Read the model definition and answer for the solid it produces. Units are mm, in the model's axes. A direction names the side the tool comes from. Give positions to 0.01 mm unless a question says otherwise; leave off trailing zeros. Loops run counter-clockwise (first coordinate to the right, second up) from the corner with the lowest first, then second, coordinate; pieces in that order, holes last. Notation, with made-up numbers: (87.5, -24.5) -> (97.5, -24.5) arc R27 ccw to (97.5, -0.5) -> close; hole circle Ø9 at (-24, -26.75). An arc over 180 degrees is marked (long way). Return JSON: item names as keys, results as strings. Group by question number.
Autodesk Inventor part; units mm, degrees
ref_plane "YZ Plane" through (0, 0, 0) normal (1, 0, 0) x (0, 1, 0)
ref_plane "XZ Plane" through (0, 0, 0) normal (0, 1, 0) x (-1, 0, 0)
ref_plane "XY Plane" through (0, 0, 0) normal (0, 0, 1) x (1, 0, 0)
sketch "Skizze1" plane through (0, 0, 0) normal (0, 0, 1) x (1, 0, 0)
  line L0 (0, 10) -> (50, 10)
  line L1 (50, 10) -> (50, -45)
  line L2 (50, -45) -> (0, -45)
  line L3 (0, -45) -> (-5, -45)
  line L4 (-5, -45) -> (-5, 10)
  line L5 (-5, 10) -> (0, 10)
  point P0 (0, 0)
  dimension "d0" = 10
  dimension "d1" = 50
  dimension "d2" = 55
  dimension "d3" = 50
  dimension "d6" = 5
extrude "Extrusion1" add sketch "Skizze1" along normal blind 3
sketch "Skizze3" plane through (0, 0, 3) normal (0, 0, 1) x (1, 0, 0)
  line L0 (50, 10) -> (-5, 10)
  line L1 (-5, 10) -> (-5, -45)
  line L2 (-5, 10) -> (-2, 10)
  line L3 (-2, 10) -> (-2, -45)
  line L4 (-5, -45) -> (50, -45)
  line L5 (-5, -45) -> (-5, 10)
  point P0 (0, 0)
  dimension "d13" = 3
extrude "Extrusion3" add sketch "Skizze3" along normal blind 20
fillet "Rundung2" radius 2 2 edges at (-2, -17.5, 3) (-5, -17.5, 0)
sketch "Skizze4" plane through (0, 0, 3) normal (0, 0, 1) x (1, 0, 0)
  circle A0 centre (46, -36.5) radius 3
  circle A1 centre (4, 6) radius 3
  circle A2 centre (4, 6) radius 1.8
  circle A3 centre (46, -36.5) radius 1.8
  point P0 (0, 0)
  dimension "d17" = 3.6
  dimension "d18" = 6
hole "Bohrung1" at (4, 6, 3) at (46, -36.5, 3) direction (0, 0, -1) diameter 6 end through all counterbore diameter 7 counterbore depth 1
properties part number "stativ"
1. Determine the mould class of faces 4 (the cylindrical face through (-1.43, -17.89, 3.6)), 5 (the flat face through (23, -17, 0)), 6 (the cylindrical face through (43.97, -34.29, 0.99)) for opening direction X: pulls with the +X half, pulls with the -X half, needs draft (parallel to the pull), parting line crosses it, or undercut.
2. Flat-ended cylindrical pins translate along their axes: pin 1 Ø4 at (x, y) = (4, 6) entering from -Z; pin 2 Ø3 at (x, y) = (8.5, -1) entering from +Z; pin 3 Ø2 at (y, z) = (-33.5, 6) entering from +X. Find the tip coordinate at first contact, or state that the pin passes through.
3. Section C-C on y = -20 is taken. Determine the outline of the cut face in (x, z), then the cut area to 3 significant figures.
4. Section B-B on x = 4 is taken. Determine the outline of the cut face in (y, z), then the cut area to 3 significant figures.
5. Straight lines are drawn through the part: line 1 (Y direction, x = 46, z = 2.5); line 2 (Y direction, x = 46, z = 0.6); line 3 (X direction, y = 6, z = 2.55). For each, find the intervals that lie inside material, in ascending order. Write a range as from..to.
6. Section D-D on z = 9.75 is taken. Determine the outline of the cut face in (x, y).
7. Section A-A on y = 6 is taken. Determine the outline of the cut face in (x, z).
8. Which of the six approach directions +Z, -Z, +X, -X, +Y, -Y give full straight-line access (tool end or side, diameter ignored) to faces 1 (the cylindrical face through (-4.4, -17.11, 0.57)), 2 (the flat face through (-2, -17, 14)), 3 (the flat face through (44, -39, 2))?
Completed:
{
 "1": {"face 4": "pulls with the +X half", "face 5": "needs draft", "face 6": "undercut"},
 "2": {"pin 1": "passes through", "pin 2": "stops at z = 3", "pin 3": "stops at x = -2"},
 "3": {"outline": "(-5, 2) arc R2 ccw to (-3, 0) -> (50, 0) -> (50, 3) -> (0, 3) arc R2 cw to (-2, 5) -> (-2, 23) -> (-5, 23) -> close", "area": "225 mm²"},
 "4": {"outline": "(-45, 0) -> (3, 0) -> (3, 2) -> (2.5, 2) -> (2.5, 3) -> (-45, 3) -> close; (9, 0) -> (10, 0) -> (10, 3) -> (9.5, 3) -> (9.5, 2) -> (9, 2) -> close", "area": "146 mm²"},
 "5": {"line 1": "y = -45..-40, -33..10", "line 2": "y = -45..-39.5, -33.5..10", "line 3": "x = -5..0.5, 7.5..50"},
 "6": {"outline": "(-5, -45) -> (-2, -45) -> (-2, 10) -> (-5, 10) -> close"},
 "7": {"outline": "(-5, 2) arc R2 ccw to (-3, 0) -> (1, 0) -> (1, 2) -> (0.5, 2) -> (0.5, 3) -> (0, 3) arc R2 cw to (-2, 5) -> (-2, 23) -> (-5, 23) -> close; (7, 0) -> (50, 0) -> (50, 3) -> (7.5, 3) -> (7.5, 2) -> (7, 2) -> close"},
 "8": {"face 1": "-Z, -X, +Y, -Y", "face 2": "+Z, +X, +Y, -Y", "face 3": "+Z"}
}
